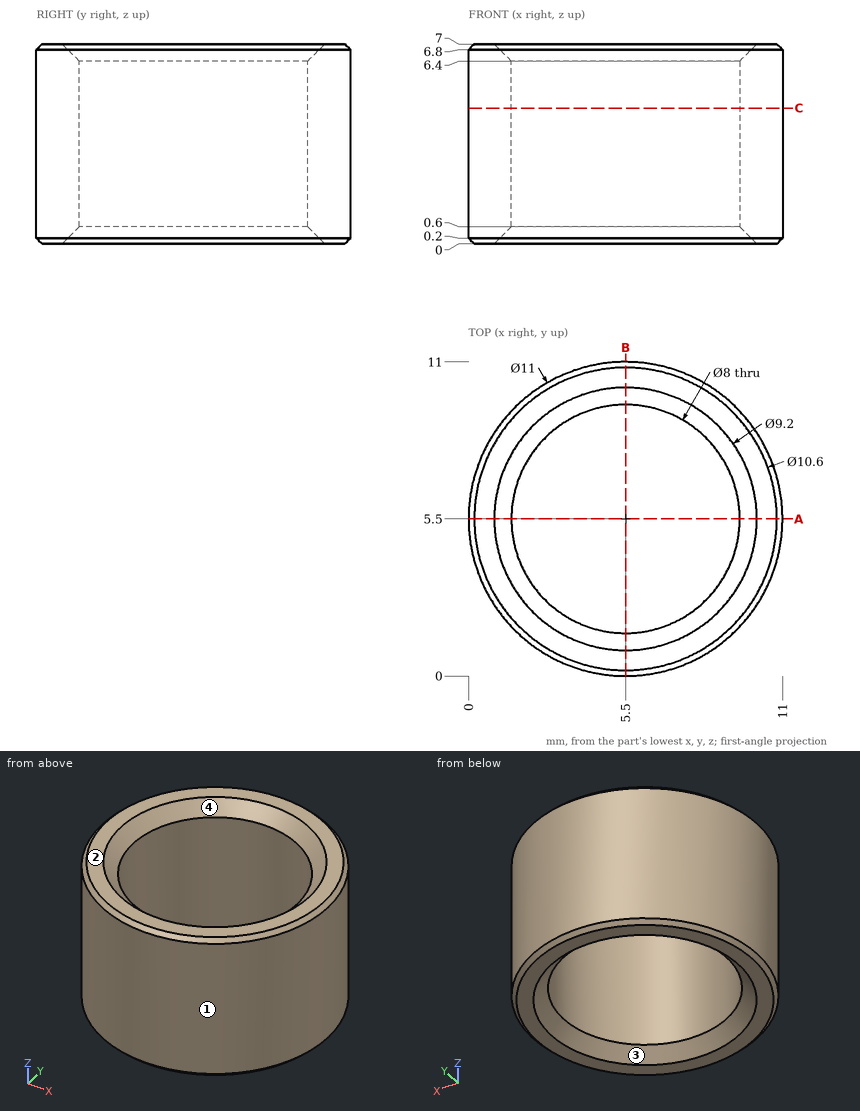
Job drawing, mm, ordinate dimensions from the low corner. One solid piece. Give positions to 0.01 mm unless a question says otherwise; leave off trailing zeros. Loops run counter-clockwise (first coordinate to the right, second up) from the corner with the lowest first, then second, coordinate; pieces in that order, holes last.
Item 1: Slice it at C-C, the plane z = 4.75. List the corners of the cut face in (x, y), and give its area (3 significant figures).
Answers follow:
outline: circle Ø11 at (5.5, 5.5); hole circle Ø8 at (5.5, 5.5)
area: 44.8 mm2
Item 2: Pull direction X, two halves, no side cores. Call the marked faces 1, 2, 3 and 4: released by +X, released by -X, zero draft, split by the parting line, or undercut.
Answers follow:
face 1: split by the parting line
face 2: zero draft
face 3: undercut
face 4: undercut
Item 3: Flat gauge pins, fed straight in: pin 1 (3 mm diameter, centred on x = 8.5, y = 9.5, fed in from -Z); pin 2 (1 mm diameter, centred on x = 2, z = 4.5, fed in from +Y); pin 3 (2 mm diameter, centred on y = 7, z = 2.5, fed in from -X); pin 4 (1 mm diameter, centred on y = 9, z = 1.5, fed in from +X). Where does each tip first touch, or does it go through?
Answers follow:
pin 1: stops at z = 0
pin 2: stops at y = 10.11
pin 3: stops at x = 0.02
pin 4: stops at x = 10.11
Item 4: Drill centre lines: line 1 (Y direction, x = 5.5, z = 3.2); line 2 (Y direction, x = 3.75, z = 5); line 3 (X direction, y = 4.5, z = 2). Where is each one in solid material? Low to high.
Answers follow:
line 1: y = 0 to 1.5, 9.5 to 11
line 2: y = 0.29 to 1.9, 9.1 to 10.71
line 3: x = 0.09 to 1.63, 9.37 to 10.91
Item 5: Slice it at A-A, the plane y = 5.5. List the corners of the cut face in (x, z).
Answers follow:
outline: (0, 0.2) - (0.2, 0) - (0.9, 0) - (1.5, 0.6) - (1.5, 6.4) - (0.9, 7) - (0.2, 7) - (0, 6.8) - close; (9.5, 0.6) - (10.1, 0) - (10.8, 0) - (11, 0.2) - (11, 6.8) - (10.8, 7) - (10.1, 7) - (9.5, 6.4) - close
